CAD build for the part. Positions are in the model's coordinates, mm. A direction names the side the tool comes from. Coordinates: 2 decimals unless noted, no trailing zeros. Loops run counter-clockwise (first coordinate to the right, second up) from the corner with the lowest first, then second, coordinate; pieces in that order, holes last.
1) Which spindle directions (+Z, -Z, +X, -X, +Y, -Y) get a long thin tool onto all of the face, cutting with end or side? Do faces 1 (the flat face through (26, 58, 20)), 2 (the flat face through (73, 55, 20)), 3 (the cylindrical face through (47.781, 65.845, 19.72)). Say none if no direction does.
2) Saw through at D-D, the plane z = 31. Write the cut outline in (x, y).
3) Two-plate mould, pull along Y, no slides. Class faces 4 (the cylindrical face through (17, 65, 22)), 5 (the flat face through (74, 59, 20)), 6 (the flat face through (24, 50, 20)), 7 (the flat face through (37, 60, 40)): +Y half, -Y half, draft (parallel to the pull), parting line (faces both ways), or undercut.
4) Saw through at C-C, the plane y = 61.5. Write the cut outline in (x, z).
5) Saw through at B-B, the plane x = 74. Write the cut outline in (y, z).
6) Pin check, flat tips, straight feed: pin 1 Ø5 at (y, z) = (65, 20) entering from +X; pin 2 Ø2 at (x, z) = (42.5, 9) entering from -Y; pin 3 Ø6.5 at (x, z) = (26.5, 9) entering from +Y. Stop position of each tip, or through.
7) Wall check: line 1 along Z through (x, y) = (26.5, 56.75); line 2 along X through (y, z) = (62.5, 37); line 3 along Y through (x, z) = (69, 19). Give the ranges that are in metal, low to high.
8) Saw through at A-A, the plane z = 20. Write the cut outline in (x, y), and give its area (3 significant figures).
```python
from build123d import *

# Parameters (mm, degrees)
SKETCH209_R     = 19
SKETCH209_R_2   = 16
PAD104_DEPTH    = 40
SKETCH210_W     = 38
SKETCH210_H     = 10
POCKET121_DEPTH = 40
SKETCH211_W     = 15
SKETCH211_H     = 4
PAD105_DEPTH    = 40
SKETCH212_R     = 2
POCKET122_DEPTH = 69.001
SKETCH213_W     = 6
SKETCH213_H     = 40
SKETCH213_W_2   = 13
SKETCH213_H_2   = 16
PAD106_DEPTH    = 40
SKETCH214_R     = 2
POCKET123_DEPTH = 6
SKETCH_W        = 90
SKETCH_H        = 30
POCKET_DEPTH    = 40.001
SKETCH215_R     = 2
POCKET124_DEPTH = 70.001


with BuildPart() as part:
    # Sketch209 → Pad104 (new body)
    with BuildSketch(Plane.XY):
        with Locations((50, 50)):
            Circle(SKETCH209_R)
        with Locations((50, 50)):
            Circle(SKETCH209_R_2, mode=Mode.SUBTRACT)
    extrude(amount=PAD104_DEPTH)

    # Sketch210 → Pocket121 (cut)
    with BuildSketch(Plane.XY):
        with Locations((69, 50)):
            Rectangle(SKETCH210_W, SKETCH210_H)
    extrude(amount=POCKET121_DEPTH, mode=Mode.SUBTRACT)

    # Sketch211 → Pad105 (join)
    with BuildSketch(Plane.XY):
        with Locations((73.5, 57)):
            Rectangle(SKETCH211_W, SKETCH211_H)
        with Locations((73.5, 43)):
            Rectangle(SKETCH211_W, SKETCH211_H)
    extrude(amount=PAD105_DEPTH)

    # Sketch212 → Pocket122 (cut, through all)
    with BuildSketch(Plane.XZ):
        with Locations((74, 31)):
            Circle(SKETCH212_R)
        with Locations((74, 9)):
            Circle(SKETCH212_R)
    extrude(amount=-POCKET122_DEPTH, mode=Mode.SUBTRACT)

    # Sketch213 → Pad106 (join)
    with BuildSketch(Plane.XY):
        with Locations((17, 50)):
            Rectangle(SKETCH213_W, SKETCH213_H)
        with Locations((26.5, 50)):
            Rectangle(SKETCH213_W_2, SKETCH213_H_2)
    extrude(amount=PAD106_DEPTH)

    # Sketch214 (on Face19 of Pad106) → Pocket123 (cut)
    with BuildSketch(Plane(origin=(14, 0, 0), x_dir=(0, -1, 0), z_dir=(-1, 0, 0))):
        with Locations((-65, 20)):
            Circle(SKETCH214_R)
        with Locations((-35, 20)):
            Circle(SKETCH214_R)
    extrude(amount=-POCKET123_DEPTH, mode=Mode.SUBTRACT)

    # Sketch → Pocket (cut, through all)
    with BuildSketch(Plane.XY):
        with Locations((48.284056, 35)):
            Rectangle(SKETCH_W, SKETCH_H)
    extrude(amount=POCKET_DEPTH, mode=Mode.SUBTRACT)

    # Sketch215 → Pocket124 (cut, through all)
    with BuildSketch(Plane.XZ):
        with Locations((26.5, 31)):
            Circle(SKETCH215_R)
        with Locations((26.5, 9)):
            Circle(SKETCH215_R)
    extrude(amount=-POCKET124_DEPTH, mode=Mode.SUBTRACT)


solid = part.part
```
Data:
1. face 1: +Z, -Z, +Y
1. face 2: +Z, -Z, +X, -Y
1. face 3: +Z, -Z, -Y
2. outline: (14, 50) - (24.5, 50) - (24.5, 58) - (20, 58) - (20, 70) - (14, 70) - close; (28.5, 50) - (34, 50) arc R16 cw to (65.2, 55) - (72, 55) - (72, 59) - (66.73, 59) arc R19 ccw to (32.77, 58) - (28.5, 58) - close; (76, 55) - (81, 55) - (81, 59) - (76, 59) - close
3. face 4: undercut
3. face 5: +Y half
3. face 6: -Y half
3. face 7: draft
4. outline: (14, 0) - (20, 0) - (20, 40) - (14, 40) - close; (34.88, 0) - (38.88, 0) - (38.88, 40) - (34.88, 40) - close; (61.12, 0) - (65.12, 0) - (65.12, 40) - (61.12, 40) - close
5. outline: (55, 0) - (59, 0) - (59, 7) - (55, 7) - close; (55, 11) - (59, 11) - (59, 29) - (55, 29) - close; (55, 33) - (59, 33) - (59, 40) - (55, 40) - close
6. pin 1: stops at x = 64.31
6. pin 2: stops at y = 63.56
6. pin 3: stops at y = 58
7. line 1: z = 0 to 7, 11 to 29, 33 to 40
7. line 2: x = 14 to 20, 35.69 to 40.01, 59.99 to 64.31
7. line 3: y = 55 to 59
8. outline: (14, 50) - (34, 50) arc R16 cw to (65.2, 55) - (81, 55) - (81, 59) - (66.73, 59) arc R19 ccw to (32.77, 58) - (20, 58) - (20, 63) - (14, 63) - close; (14, 67) - (20, 67) - (20, 70) - (14, 70) - close
8. area: 392 mm2
